```python
from build123d import *

# Parameters (mm, degrees)
CROQUIS1_W              = 29
CROQUIS1_H              = 28
SALIENTE_EXTRUIR1_DEPTH = 23
CROQUIS2_W              = 23
CROQUIS2_H              = 20
CORTAR_EXTRUIR1_DEPTH   = 25
SALIENTE_EXTRUIR5_DEPTH = 5
CROQUIS12_R             = 1
SALIENTE_EXTRUIR7_DEPTH = 0.75
CROQUIS13_R             = 1.5
CROQUIS13_W             = 5
CROQUIS13_H             = 5
SALIENTE_EXTRUIR8_DEPTH = 3


with BuildPart() as part:
    # Croquis1 → Saliente-Extruir1 (new body)
    with BuildSketch(Plane(origin=(0, 0, 0), x_dir=(1, 0, 0), z_dir=(0, 1, 0))):
        Rectangle(CROQUIS1_W, CROQUIS1_H)
    extrude(amount=SALIENTE_EXTRUIR1_DEPTH)

    # Croquis2 → Cortar-Extruir1 (cut)
    with BuildSketch(Plane.XY.offset(14)):
        with Locations((0, 10)):
            Rectangle(CROQUIS2_W, CROQUIS2_H)
    extrude(amount=-CORTAR_EXTRUIR1_DEPTH, mode=Mode.SUBTRACT)

    # Croquis10 → Saliente-Extruir5 (add)
    with BuildSketch(Plane.XZ):
        with BuildLine():
            Line((11.5, 14), (14.5, 14))
            Line((14.5, 14), (14.5, 15.5))
            ThreePointArc((14.5, 15.5), (13, 17), (11.5, 15.5))
            Line((11.5, 15.5), (11.5, 14))
        make_face()
    saliente_extruir5 = extrude(amount=-SALIENTE_EXTRUIR5_DEPTH)

    # Croquis12 → Saliente-Extruir7 (add)
    with BuildSketch(Plane(origin=(0, 5, 0), x_dir=(1, 0, 0), z_dir=(0, 1, 0))):
        with Locations(Location((13, -15.5, 0), (0, 0, 90))):
            Circle(CROQUIS12_R)
    saliente_extruir7 = extrude(amount=SALIENTE_EXTRUIR7_DEPTH)

    # Simetría1: Saliente-Extruir5, Saliente-Extruir7 across plane
    add(saliente_extruir5.mirror(Plane(origin=(0, 10, 0), x_dir=(0, 0, 1), z_dir=(0, -1, 0))))
    add(saliente_extruir7.mirror(Plane(origin=(0, 10, 0), x_dir=(0, 0, 1), z_dir=(0, -1, 0))))

    # Croquis13 → Saliente-Extruir8 (add)
    # profile 1 of 2: a face of its own
    with BuildSketch(Plane.XY.offset(14)):
        Polygon((18, 12.5), (23, 12.5), (23, 7.5), (18, 7.5), (14.5, 7.5), (14.5, 12.5), align=None)
        with Locations((20.5, 10)):
            Circle(CROQUIS13_R, mode=Mode.SUBTRACT)
    # profile 2 of 2: a face of its own
    with BuildSketch(Plane.XY.offset(14)):
        with Locations((-17, 10)):
            Rectangle(CROQUIS13_W, CROQUIS13_H)
        with Locations((-17, 10)):
            Circle(CROQUIS13_R, mode=Mode.SUBTRACT)
    extrude(amount=-SALIENTE_EXTRUIR8_DEPTH)


solid = part.part
```
Source: CAD feature listing. Evaluate the final solid. Frame: model axes, mm. A direction names the side the tool comes from. Round coordinates to 2 decimals unless told otherwise and drop trailing zeros. Loops run counter-clockwise (first coordinate to the right, second up) from the corner with the lowest first, then second, coordinate; pieces in that order, holes last. Notation, with made-up numbers: M 54.5,59 L 78.5,59 A6 cw 78.5,69 Z; hole C -1.75,55.5 d11. An arc over 180 degrees is marked long. Use a Markdown table: item, result. Add a question column.
1. Contact query for flat-ended pins moving along their axis: pin 1 (5.5 mm diameter, centred on x = 20, y = 9.5, fed in from -Z); pin 2 (11.5 mm diameter, centred on x = -7, y = 11.5, fed in from +Z); pin 3 (5 mm diameter, centred on y = 13, z = 5.5, fed in from -X); pin 4 (3.5 mm diameter, centred on x = 13.5, z = 15, fed in from +Y). Output: stop coordinate, or through.
2. Cut plane C-C, the plane z = 13. Output: boundary loops of the cut face in (x, y).
3. Pull-direction query (X, two-part tool) for faces 1 (the flat face through (23, 10, 13)), 2 (the flat face through (0, 11, -14)), 3 (the flat face through (0, 10, -11)); classes: +X half, -X half, draft (parallel to the pull), parting line (faces both ways), or undercut.
4. Cut plane B-B, the plane x = 20.5. Output: boundary loops of the cut face in (y, z).
5. Cut plane A-A, the plane y = 10. Output: boundary loops of the cut face in (x, z), and give its area (4 significant figures).
6. Cut plane D-D, the plane x = 13. Output: boundary loops of the cut face in (y, z).
7. Set-up query: faces 4 (the flat face through (-17, 12.5, 13)), 5 (the flat face through (0, 20, 2)), 6 (the flat face through (13, 14.25, 16)), 7 (the flat face through (18.8, 10, 11)), 8 (the flat face through (19, 7.5, 13)). Return all of +Z, -Z, +X, -X, +Y, -Y with unobstructed straight access to the full face (end or side cutting, diameter ignored); none if empty.
8. Ray query, line 1 along X through (y, z) = (10.5, 5); line 2 along Y through (x, z) = (-17, 12.7); line 3 along Z through (x, y) = (-8.5, 2.75). Return the intervals inside material, ascending. Write a range as [from, to].
Solution:
| question | item | result |
|---|---|---|
| 1 | pin 1 | stops at z = 11 |
| 1 | pin 2 | stops at z = 14 |
| 1 | pin 3 | stops at x = -14.5 |
| 1 | pin 4 | stops at y = 23 |
| 2 | outline | M -19.5,7.5 L -14.5,7.5 L -14.5,0 L -11.5,0 L -11.5,20 L 11.5,20 L 11.5,0 L 14.5,0 L 14.5,7.5 L 23,7.5 L 23,12.5 L 14.5,12.5 L 14.5,23 L -14.5,23 L -14.5,12.5 L -19.5,12.5 Z; hole C -17,10 d3; hole C 20.5,10 d3 |
| 3 | face 1 | +X half |
| 3 | face 2 | draft |
| 3 | face 3 | undercut |
| 4 | outline | M 7.5,11 L 8.5,11 L 8.5,14 L 7.5,14 Z; M 11.5,11 L 12.5,11 L 12.5,14 L 11.5,14 Z |
| 5 | outline | M -19.5,11 L -18.5,11 L -18.5,14 L -19.5,14 Z; M -15.5,11 L -14.5,11 L -14.5,-14 L 14.5,-14 L 14.5,11 L 19,11 L 19,14 L 11.5,14 L 11.5,-11 L -11.5,-11 L -11.5,14 L -15.5,14 Z; M 22,11 L 23,11 L 23,14 L 22,14 Z |
| 5 | area | 259.5 mm2 |
| 6 | outline | M 0,-14 L 23,-14 L 23,14 L 20,14 L 20,17 L 15,17 L 15,16.5 L 14.25,16.5 L 14.25,14.5 L 15,14.5 L 15,14 L 5,14 L 5,14.5 L 5.75,14.5 L 5.75,16.5 L 5,16.5 L 5,17 L 0,17 Z |
| 7 | face 4 | +Z, -Z, -X, +Y |
| 7 | face 5 | +Z, -Y |
| 7 | face 6 | +Z, +X, -X |
| 7 | face 7 | -Z, +X, +Y, -Y |
| 7 | face 8 | +Z, -Z, +X, -Y |
| 8 | line 1 | x = [-14.5, -11.5], [11.5, 14.5] |
| 8 | line 2 | y = [7.5, 8.5], [11.5, 12.5] |
| 8 | line 3 | z = [-14, -11] |
